Work out the finished part from the listing and answer in its coordinate system (mm). A direction names the side the tool comes from. Coordinates: 2 decimals unless noted, no trailing zeros. Order: outer loops, then holes, each group sorted by start corner. A loop starts at its lowest first (then second) coordinate and runs counter-clockwise, first axis right, second up.
1. Find the intervals of material crossed by probe 1 along Z at (x, y) = (3.4, -31.75); probe 2 along Z at (x, y) = (5.5, -10); probe 3 along Y at (x, z) = (0.75, 0), in increasing order.
2. The part is cut by section A-A, the plane y = -31.75. Give the vertices of the cut face in (x, z), then the cut area to 3 significant figures.
3. The part is cut by section B-B, the plane z = 6. Give the vertices of the cut face in (x, y).
4. A flat-ended cylindrical pin translates along its axis: pin 1 Ø6.5 at (y, z) = (60.5, -27.5) entering from +X. Find the tip coordinate at first contact, or state that the pin passes through.
5. A tool of negligible diameter and unlimited length cuts with its end or side. For faces 5 (the flat face through (3.131, 57.246, -1.919)), 6 (the flat face through (5.08, -30, 22)), from which of +Z, -Z, +X, -X, +Y, -Y can it reach the whole face along a straight path? Write none if from no direction.
6. The part is cut by section D-D, the plane z = 19. Give the vertices of the cut face in (x, y).
7. The part is cut by section C-C, the plane x = 1. Give the vertices of the cut face in (y, z) (3 decimals).
8. Determine the mould class of faces 1 (the cylindrical face through (3.219, -76.949, -37.256)), 2 (the flat face through (5.08, 63, -30)), 3 (the flat face through (3.1, -59.2, -1.3)), 4 (the cylindrical face through (5.724, -54.336, -32.533)) for opening direction Z: +Z half, -Z half, draft (parallel to the pull), parting line (faces both ways), or undercut.
```python
from build123d import *

# Parameters (mm, degrees)
SKETCH2_R           = 3.175
SKETCH2_R_2         = 9.525
BOSS_EXTRUDE1_DEPTH = 6.35
SKETCH3_R           = 6.35
CUT_EXTRUDE1_DEPTH  = 1.27
FILLET1_R           = 6.35


with BuildPart() as part:
    # Sketch2 → Boss-Extrude1 (new body)
    with BuildSketch(Plane(origin=(0, 0, 0), x_dir=(0, 0, -1), z_dir=(1, 0, 0))):
        Polygon((-30.570599259, 35.964413408), (-30.570599259, -40.235586592), (40.549400741, -82.55), (40.549400741, 82.55), align=None)
        with Locations((29.119400741, 59.69)):
            Circle(SKETCH2_R, mode=Mode.SUBTRACT)
        with Locations((-19.140599259, 30.292732622)):
            Circle(SKETCH2_R, mode=Mode.SUBTRACT)
        with Locations((29.119400741, -59.69)):
            Circle(SKETCH2_R, mode=Mode.SUBTRACT)
        with Locations((-19.140599259, -31.75)):
            Circle(SKETCH2_R, mode=Mode.SUBTRACT)
        with Locations((-5.170599259, -6.35)):
            Circle(SKETCH2_R_2, mode=Mode.SUBTRACT)
    extrude(amount=BOSS_EXTRUDE1_DEPTH)

    # Sketch3 → Cut-Extrude1 (cut)
    with BuildSketch(Plane(origin=(6.35, 0, 0), x_dir=(0, 0, -1), z_dir=(1, 0, 0))):
        with Locations((-19.140599259, 30.292732622)):
            Circle(SKETCH3_R)
        with Locations((29.119400741, 59.69)):
            Circle(SKETCH3_R)
        with Locations((-19.140599259, -31.75)):
            Circle(SKETCH3_R)
        with Locations((29.119400741, -59.69)):
            Circle(SKETCH3_R)
    extrude(amount=-CUT_EXTRUDE1_DEPTH, mode=Mode.SUBTRACT)

    # Fillet1
    fillet1_edges = [part.edges().sort_by_distance(p)[0] for p in [
        (3.175, 82.55, -40.549400741),
        (3.175, -82.55, -40.549400741),
        (3.175, -40.235586592, 30.570599259),
        (3.175, 35.964413408, 30.570599259),
    ]]
    fillet(fillet1_edges, radius=FILLET1_R)


solid = part.part
```
Geometry says:
1. probe 1: z = -40.55 to 15.97, 22.32 to 30.57
1. probe 2: z = -40.55 to -3.63, 13.97 to 30.57
1. probe 3: y = -58.42 to -14.35, 1.65 to 55.99
2. outline: (0, -40.55) - (6.35, -40.55) - (6.35, 12.79) - (5.08, 12.79) - (5.08, 15.97) - (0, 15.97) - close; (0, 22.32) - (5.08, 22.32) - (5.08, 25.49) - (6.35, 25.49) - (6.35, 30.57) - (0, 30.57) - close
2. area: 403 mm2
3. outline: (0, -54.85) - (6.35, -54.85) - (6.35, -15.84) - (0, -15.84) - close; (0, 3.14) - (6.35, 3.14) - (6.35, 52.06) - (0, 52.06) - close
4. pin 1: stops at x = 5.08
5. face 5: +Z, +X, -X, +Y
5. face 6: +X
6. outline: (0, -47.12) - (6.35, -47.12) - (6.35, -38.1) - (5.08, -38.1) - (5.08, -34.92) - (0, -34.92) - close; (0, -28.58) - (5.08, -28.58) - (5.08, -25.4) - (6.35, -25.4) - (6.35, 23.94) - (5.08, 23.94) - (5.08, 27.12) - (0, 27.12) - close; (0, 33.46) - (5.08, 33.46) - (5.08, 36.64) - (6.35, 36.64) - (6.35, 43.54) - (0, 43.54) - close
7. outline: (-76.84, -30.953) arc R6.35 ccw to (-71.383, -40.549) - (70.8, -40.549) arc R6.35 ccw to (76.111, -30.72) - (37.845, 27.7) arc R6.35 ccw to (32.533, 30.571) - (-36.625, 30.571) arc R6.35 ccw to (-42.082, 27.467) - close; hole circle Ø6.35 at (-59.69, -29.119); hole circle Ø6.35 at (-31.75, 19.141); hole circle Ø19.05 at (-6.35, 5.171); hole circle Ø6.35 at (30.293, 19.141); hole circle Ø6.35 at (59.69, -29.119)
8. face 1: parting line
8. face 2: undercut
8. face 3: +Z half
8. face 4: undercut
